Read the model definition and answer for the solid it produces. Units are mm, in the model's axes. A direction names the side the tool comes from. Give positions to 0.01 mm unless a question says otherwise; leave off trailing zeros. Order: outer loops, then holes, each group sorted by start corner. A loop starts at its lowest first (then second) coordinate and runs counter-clockwise, first axis right, second up. Notation, with made-up numbers: (-22.5, 77.5) -> (17.5, 77.5) arc R20 ccw to (17.5, 112.5) -> close; hole circle Ø7 at (-30, 32.5). An arc over 180 degrees is marked (long way). Use one line per item in the form item = value.
```python
from build123d import *

# Parameters (mm, degrees)
F0_R          = 60
F0_R_2        = 6
F0_R_3        = 40
F1_DEPTH      = 10
F2_R          = 41.5
F2_R_2        = 40
F3_DEPTH      = 250
F4_R          = 15
F5_DEPTH      = 70.8
F5_DEPTH_BACK = 74.6


with BuildPart() as f1:
    # F0 (on Front) → F1 (new body)
    with BuildSketch(Plane.XZ):
        Circle(F0_R)
        with Locations((-44.167295593, -25.5)):
            Circle(F0_R_2, mode=Mode.SUBTRACT)
        with Locations((0, -51)):
            Circle(F0_R_2, mode=Mode.SUBTRACT)
        with Locations((44.167295593, -25.5)):
            Circle(F0_R_2, mode=Mode.SUBTRACT)
        with Locations((-44.167295593, 25.5)):
            Circle(F0_R_2, mode=Mode.SUBTRACT)
        Circle(F0_R_3, mode=Mode.SUBTRACT)
        with Locations((44.167295593, 25.5)):
            Circle(F0_R_2, mode=Mode.SUBTRACT)
        with Locations((0, 51)):
            Circle(F0_R_2, mode=Mode.SUBTRACT)
    extrude(amount=F1_DEPTH)

    # F2 (on face) → F3 (join)
    with BuildSketch(Plane.XZ.offset(10)):
        Circle(F2_R)
        Circle(F2_R_2, mode=Mode.SUBTRACT)
    extrude(amount=F3_DEPTH)

    # F4 (on Top) → F5 (cut, two sides)
    with BuildSketch(Plane.XY) as f5_sk:
        with Locations((0, -98)):
            Circle(F4_R)
    extrude(amount=-F5_DEPTH, mode=Mode.SUBTRACT)
    extrude(f5_sk.sketch, amount=F5_DEPTH_BACK, mode=Mode.SUBTRACT)


solid = f1.part
```
Item 1: Given pin 1 Ø8 at (x, y) = (37, -68) entering from -Z; pin 2 Ø12 at (x, y) = (-26.5, -102) entering from -Z; pin 3 Ø10 at (x, z) = (-36.5, 45) entering from -Y; pin 4 Ø7 at (x, z) = (0, -51) entering from -Y, each flat-ended and moving along its own axis, determine where each tip first touches the part or whether it passes through.
Checks:
pin_1 = -25.16
pin_2 = -36.08
pin_3 = -10
pin_4 = through
Item 2: Which of the six approach directions +Z, -Z, +X, -X, +Y, -Y give full straight-line access (tool end or side, diameter ignored) to faces 4 (the cylindrical face through (7.69, -85.12, 39.77)), 5 (the cylindrical face through (39.584, -133.25, 12.465))?
Checks:
face_4 = +Z, -Z
face_5 = -Y
Item 3: The part is cut by section D-D on z = 11. Give the vertices of the cut face in (x, y), and give its area (3 significant figures).
Checks:
outline = (-58.98, -10) -> (-40.02, -10) -> (-40.02, -260) -> (-38.46, -260) -> (-38.46, 0) -> (-58.98, 0) -> close; (38.46, -260) -> (40.02, -260) -> (40.02, -10) -> (58.98, -10) -> (58.98, 0) -> (38.46, 0) -> close
area = 1,190 mm²
Item 4: The part is cut by section C-C on y = -98. Give the vertices of the cut face in (x, z), and give its area (3 significant figures).
Checks:
outline = (-15, -38.69) -> (-15, -37.08) arc R40 cw to (-15, 37.08) -> (-15, 38.69) arc R41.5 ccw to start; (15, -38.69) arc R41.5 ccw to (15, 38.69) -> (15, 37.08) arc R40 cw to (15, -37.08) -> close
area = 292 mm²
Item 5: Straight lines are drawn through the part: L1, parallel to Z at x = 0, y = -5; L2, parallel to Z at x = 0, y = -76.5; L3, parallel to X at y = -50, z = 1.5. For each, find the intervals that lie inside material, in ascending order. Write a range as from..to.
Checks:
L1 = -60..-57, -45..-40, 40..45, 57..60
L2 = -41.5..-40, 40..41.5
L3 = -41.47..-39.97, 39.97..41.47
Item 6: The part is cut by section A-A on x = 0. Give the vertices of the cut face in (y, z).
Checks:
outline = (-260, -41.5) -> (-113, -41.5) -> (-113, -40) -> (-260, -40) -> close; (-260, 40) -> (-113, 40) -> (-113, 41.5) -> (-260, 41.5) -> close; (-83, -41.5) -> (-10, -41.5) -> (-10, -45) -> (0, -45) -> (0, -40) -> (-83, -40) -> close; (-83, 40) -> (0, 40) -> (0, 45) -> (-10, 45) -> (-10, 41.5) -> (-83, 41.5) -> close; (-10, -60) -> (0, -60) -> (0, -57) -> (-10, -57) -> close; (-10, 57) -> (0, 57) -> (0, 60) -> (-10, 60) -> close
Item 7: The part is cut by section B-B on z = 25.5. Give the vertices of the cut face in (x, y), and give its area (3 significant figures).
Checks:
outline = (-54.31, -10) -> (-50.17, -10) -> (-50.17, 0) -> (-54.31, 0) -> close; (-38.17, -10) -> (-32.74, -10) -> (-32.74, -260) -> (-30.82, -260) -> (-30.82, 0) -> (-38.17, 0) -> close; (30.82, -260) -> (32.74, -260) -> (32.74, -10) -> (38.17, -10) -> (38.17, 0) -> (30.82, 0) -> close; (50.17, -10) -> (54.31, -10) -> (54.31, 0) -> (50.17, 0) -> close
area = 1,190 mm²
Item 8: Determine the mould class of faces 1 (the cylindrical face through (-59.94, -4.93, 2.64)), 2 (the cylindrical face through (7.69, -85.12, -39.77)), 3 (the flat face through (-22, -260, 34)) for opening direction X: +X half, -X half, draft (parallel to the pull), parting line (faces both ways), or undercut.
Checks:
face_1 = parting line
face_2 = undercut
face_3 = draft
